Part model, mm, in its own coordinate system. A direction names the side the tool comes from. Round coordinates to 2 decimals unless told otherwise and drop trailing zeros. Write each loop counter-clockwise with the first axis right and the second up, starting at its lowest first coordinate (ties: lowest second). Pieces come first, ordered by that corner, then holes.
1) Which spindle directions (+Z, -Z, +X, -X, +Y, -Y) get a long thin tool onto all of the face, cutting with end or side? Do faces 1 (the flat face through (-2, 28, 1)), 2 (the flat face through (15, 6, 1)), 3 (the flat face through (-2, 14, 1)). Say none if no direction does.
2) Flat gauge pins, fed straight in: pin 1 (1.5 mm diameter, centred on y = 9, z = 1, fed in from -X); pin 2 (1.5 mm diameter, centred on y = 5, z = 1.5, fed in from +X); pin 3 (0.9 mm diameter, centred on x = 33, z = 1.5, fed in from +Y). Where does each tip first touch, or does it go through?
3) Drill centre lines: L1, parallel to Y at x = 19, z = 1.7; L2, parallel to X at y = 37.5, z = 1.65. Where is each one in solid material? Low to high.
4) Saw through at B-B on z = 1.25. Write the cut outline in (x, y).
5) Pull direction Y, two halves, no side cores. Call faces 4 (the flat face through (15, 21, 3)), 5 (the flat face through (20.67, 4, 1)), 6 (the flat face through (15, 42, 1)): +Y half, -Y half, draft (parallel to the pull), parting line (faces both ways), or undercut.
6) Saw through at C-C on y = 35. Write the cut outline in (x, z).
7) Saw through at A-A on x = 14.5. Write the cut outline in (y, z).
```python
from build123d import *

# Parameters (mm, degrees)
ESQUISSE1_W        = 31
ESQUISSE1_H        = 42
ESQUISSE1_W_2      = 10.34
ESQUISSE1_H_2      = 3
ESQUISSE1_W_3      = 3
ESQUISSE1_H_3      = 14
BOSS_EXTRU_1_DEPTH = 3


with BuildPart() as part:
    # Esquisse1 → Boss.-Extru.1 (new body)
    # profile 1 of 3: a face of its own
    with BuildSketch(Plane.XY):
        with Locations((15.5, 21)):
            Rectangle(ESQUISSE1_W, ESQUISSE1_H)
        with Locations((15.5, 4.5)):
            Rectangle(ESQUISSE1_W_2, ESQUISSE1_H_2, mode=Mode.SUBTRACT)
    # profile 2 of 3: a face of its own
    with BuildSketch(Plane.XY):
        with Locations((-1.5, 21)):
            Rectangle(ESQUISSE1_W_3, ESQUISSE1_H_3)
    # profile 3 of 3: a face of its own
    with BuildSketch(Plane.XY):
        with Locations((32.5, 21)):
            Rectangle(ESQUISSE1_W_3, ESQUISSE1_H_3)
    extrude(amount=BOSS_EXTRU_1_DEPTH)


solid = part.part
```
Completed:
1. face 1: +Z, -Z, -X, +Y
1. face 2: +Z, -Z
1. face 3: +Z, -Z, -X, -Y
2. pin 1: stops at x = 0
2. pin 2: stops at x = 31
2. pin 3: stops at y = 28
3. L1: y = 0 to 3, 6 to 42
3. L2: x = 0 to 31
4. outline: (-3, 14) - (0, 14) - (0, 0) - (31, 0) - (31, 14) - (34, 14) - (34, 28) - (31, 28) - (31, 42) - (0, 42) - (0, 28) - (-3, 28) - close; hole (10.33, 3) - (20.67, 3) - (20.67, 6) - (10.33, 6) - close
5. face 4: draft
5. face 5: undercut
5. face 6: +Y half
6. outline: (0, 0) - (31, 0) - (31, 3) - (0, 3) - close
7. outline: (0, 0) - (3, 0) - (3, 3) - (0, 3) - close; (6, 0) - (42, 0) - (42, 3) - (6, 3) - close
